from build123d import *

# Parameters (mm, degrees)
SKETCH1_R           = 2.1
SKETCH1_R_2         = 2.2
BOSS_EXTRUDE1_DEPTH = 5
SKETCH2_R           = 1.4
CUT_EXTRUDE1_DEPTH  = 6


with BuildPart() as part:
    # Sketch1 → Boss-Extrude1 (new body)
    with BuildSketch(Plane.XY):
        with BuildLine():
            Line((41, 136.6), (41, 125.6))
            ThreePointArc((41, 125.6), (41.878679656, 123.478679656), (44, 122.6))
            Line((44, 122.6), (47, 122.6))
            Line((47, 122.6), (47, -29.8))
            Line((47, -29.8), (47, -58.8))
            Line((47, -58.8), (43.5, -58.8))
            Line((43.5, -58.8), (43.5, -63.8))
            Line((43.5, -63.8), (10, -63.8))
            Line((10, -63.8), (10, -29.8))
            Line((10, -29.8), (10, -12.5))
            Line((10, -12.5), (0, -12.5))
            ThreePointArc((0, -12.5), (-12.5, 0), (0, 12.5))
            Line((0, 12.5), (16, 12.5))
            Line((16, 12.5), (16, 104.5))
            Line((16, 104.5), (0, 104.5))
            ThreePointArc((0, 104.5), (-8.838834765, 108.161165235), (-12.5, 117))
            Line((-12.5, 117), (-12.5, 124.1))
            ThreePointArc((-12.5, 124.1), (-8.838834765, 132.938834765), (0, 136.6))
            Line((0, 136.6), (0, 174))
            Line((0, 174), (2.5, 174))
            ThreePointArc((2.5, 174), (6.035533906, 175.464466094), (7.5, 179))
            ThreePointArc((7.5, 179), (12.5, 184), (17.5, 179))
            ThreePointArc((17.5, 179), (18.964466094, 175.464466094), (22.5, 174))
            Line((22.5, 174), (37.5, 174))
            Line((37.5, 174), (37.5, 136.6))
            Line((37.5, 136.6), (41, 136.6))
        make_face()
        Circle(SKETCH1_R, mode=Mode.SUBTRACT)
        with Locations((0, 117)):
            Circle(SKETCH1_R, mode=Mode.SUBTRACT)
        with Locations((12.5, 179)):
            Circle(SKETCH1_R_2, mode=Mode.SUBTRACT)
    extrude(amount=BOSS_EXTRUDE1_DEPTH)

    # Sketch2 → Cut-Extrude1 (cut, through all)
    with BuildSketch(Plane.XY.offset(5)):
        with Locations((13.2, -21.3)):
            Circle(SKETCH2_R)
        with Locations((24.5, 134)):
            Circle(SKETCH2_R)
    extrude(amount=-CUT_EXTRUDE1_DEPTH, mode=Mode.SUBTRACT)


solid = part.part
Verification items for the finished model (mm, model axes). A direction names the side the tool comes from. Coordinates: 2 decimals unless noted, no trailing zeros. Loops run counter-clockwise (first coordinate to the right, second up) from the corner with the lowest first, then second, coordinate; pieces in that order, holes last. Notation, with made-up numbers: (47.25, 11) -> (93.25, 11) arc R7 ccw to (93.25, 16) -> close; hole circle Ø11 at (17, 58). An arc over 180 degrees is marked (long way). Answer as a JSON object with one key per item and string values. Group by question number.
Item 1: Sectioned sample at D-D on x = 28.5. Record the boundary of the cut face in (y, z).
Item 2: Sectioned sample at B-B on x = -7. Record the boundary of the cut face in (y, z), plus the area to 3 significant figures.
Item 3: Tool access check on faces 5 (the flat face through (0, 155, 2)), 6 (the flat face through (41, 131, 2)), 7 (the flat face through (5, -12.5, 2)), 8 (the flat face through (16, 58, 2)), 9 (the flat face through (47, 33, 2)). Record the directions out of +Z, -Z, +X, -X, +Y, -Y that give a thin tool (end or side, any length) a straight path to the whole face; none if there is none.
Item 4: Sectioned sample at A-A on z = 2.3. State how many separate pieces and enclosed holes the cut face has, plus the area to 3 significant figures.
Item 5: Scan lines: probe 1 along Y at (x, z) = (1, 3.15); probe 2 along Y at (x, z) = (24.5, 3.95); probe 3 along Y at (x, z) = (12.5, 1.95). Record each from-to range of solid material in increasing order.
Item 6: Depth check by flat-ended pin: pin 1 (1.8 mm diameter, centred on x = 39, z = 1.5, fed in from +Y); pin 2 (1 mm diameter, centred on x = 23, z = 2.5, fed in from +Y); pin 3 (2.5 mm diameter, centred on x = 13.2, y = -21.3, fed in from +Z); pin 4 (1.8 mm diameter, centred on x = 45, z = 3, fed in from -Y). Enter the tip coordinate at first touch or a pass-through.
Item 7: Mould release check, pull along Y, two halves, no side actions. Record for faces 1 (the flat face through (24, 62, 5)), 2 (the cylindrical face through (2.003, 0.631, 2.465)), 3 (the flat face through (8, 12.5, 2)), 4 (the flat face through (27, -63.8, 2)): +Y half, -Y half, draft (parallel to the pull), parting line (faces both ways), or undercut.
Item 8: Sectioned sample at C-C on y = 56. Record the boundary of the cut face in (x, z).
Evaluation:
{
 "1": {"outline": "(-63.8, 0) -> (174, 0) -> (174, 5) -> (-63.8, 5) -> close"},
 "2": {"outline": "(-10.36, 0) -> (10.36, 0) -> (10.36, 5) -> (-10.36, 5) -> close; (106.64, 0) -> (134.46, 0) -> (134.46, 5) -> (106.64, 5) -> close", "area": "243 mm²"},
 "3": {"face 5": "+Z, -Z, -X, +Y", "face 6": "+Z, -Z, +X, +Y", "face 7": "+Z, -Z, -X, -Y", "face 8": "+Z, -Z, -X", "face 9": "+Z, -Z, +X, +Y, -Y"},
 "4": {"separate pieces": "1", "enclosed holes": "5", "area": "9,360 mm²"},
 "5": {"probe 1": "y = -12.5 to -1.85, 1.85 to 12.5, 104.5 to 115.15, 118.85 to 174", "probe 2": "y = -63.8 to 132.6, 135.4 to 174", "probe 3": "y = -63.8 to -22.51, -20.09 to 12.5, 104.5 to 176.8, 181.2 to 184"},
 "6": {"pin 1": "stops at y = 136.6", "pin 2": "stops at y = 174", "pin 3": "passes through", "pin 4": "stops at y = -58.8"},
 "7": {"face 1": "draft", "face 2": "undercut", "face 3": "undercut", "face 4": "-Y half"},
 "8": {"outline": "(16, 0) -> (47, 0) -> (47, 5) -> (16, 5) -> close"}
}
